Verification items for the finished model (mm, model axes). Face numbers are marked on the shaded views. A direction names the side the tool comes from. Round coordinates to 2 decimals unless told otherwise and drop trailing zeros. Order: outer loops, then holes, each group sorted by start corner. A loop starts at its lowest first (then second) coordinate and runs counter-clockwise, first axis right, second up. Notation, with made-up numbers: M -8.5,-17 L 45.5,-17 A36 cw 45.5,17 Z; hole C 10,74.25 d3. An arc over 180 degrees is marked long. Use CSV: the item, a comma, the result in double quotes. Start each with the question number.
Q1. Set-up check for the marked faces 1 and 2: record each of +Z, -Z, +X, -X, +Y, -Y from which the full face is reachable in a straight line by a thin tool's end or side.
Q2. Mould release check, pull along Y, two halves, no side actions. Record for the marked faces 3, 4, 5 and 6: +Y half, -Y half, draft (parallel to the pull), parting line (faces both ways), or undercut.
Q3. Scan lines: line 1 (Y direction, x = -143.5, z = -31.35); line 2 (Y direction, x = -143.5, z = -35.2); line 3 (X direction, y = 87, z = -26). Record each from-to range of solid material in increasing order.
Q4. Gauge pin test, flat ends, axial feed: pin 1 Ø1.5 at (y, z) = (127, -5.5) entering from +X; pin 2 Ø2 at (x, z) = (-37.5, -16.5) entering from -Y; pin 3 Ø4 at (x, y) = (-32.5, 143.5) entering from -Z. Record the tip position at first contact, or that the pin passes through.
Q5. Sectioned sample at A-A (z = -9.5). Enter the section's corners in (x, y), and give its area (3 significant figures).
Q6. Sectioned sample at B-B (y = 44). Enter the section's corners in (x, z).
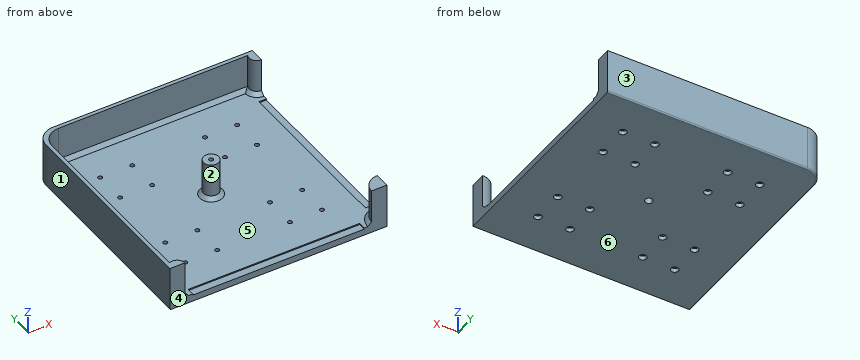
```python
from build123d import *

# Parameters (mm, degrees)
PAD005_DEPTH         = 6.25
SKETCH009_R          = 6.25
PAD006_DEPTH         = 30
SKETCH010_R          = 1.75
POCKET002_DEPTH      = 100
POCKET002_DEPTH_BACK = 100
SKETCH011_R          = 3
POCKET003_DEPTH      = 3.25
CHAMFER003_SIZE      = 3
FILLET003_R          = 1
SKETCH012_W          = 6
SKETCH012_H          = 139
SKETCH012_W_2        = 139
SKETCH012_H_2        = 6
POCKET004_DEPTH      = 1
SKETCH019_R          = 3
POCKET008_DEPTH      = 100
POCKET008_DEPTH_BACK = 24
SKETCH020_R          = 1.75
POCKET009_DEPTH      = 100
POCKET009_DEPTH_BACK = 100


with BuildPart() as part:
    # Sketch008 → Pad005 (new body)
    with BuildSketch(Plane.XY):
        with BuildLine():
            Line((88, 88), (-73.833333, 88))
            ThreePointArc((-73.833333, 88), (-83.850679, 83.850679), (-88, 73.833333))
            Line((-88, 73.833333), (-88, -88))
            Line((-88, -88), (88, -88))
            Line((88, -88), (88, 88))
        make_face()
    extrude(amount=-PAD005_DEPTH)

    # Sketch009 → Pad006 (join)
    with BuildSketch(Plane.XY):
        Circle(SKETCH009_R)
        with BuildLine():
            Line((-88, -88), (-88, 73.833333))
            ThreePointArc((-73.833333, 88), (-83.850679, 83.850679), (-88, 73.833333))
            Line((-73.833333, 88), (88, 88))
            Line((88, 88), (88, 75.889985))
            ThreePointArc((82.442769, 85), (82.664384, 78.885188), (88, 75.889985))
            Line((-70.83277, 85), (82.442769, 85))
            ThreePointArc((-70.83277, 85), (-80.85048, 80.850878), (-85, 70.833333))
            Line((-85, -82.408681), (-85, 70.833333))
            ThreePointArc((-75.957213, -88), (-78.920301, -82.684108), (-85, -82.408681))
            Line((-88, -88), (-75.957213, -88))
        make_face()
        with BuildLine():
            ThreePointArc((88, -75.5), (79.161165, -79.161165), (75.5, -88))
            Line((88, -88), (75.5, -88))
            Line((88, -88), (88, -75.5))
        make_face()
    extrude(amount=PAD006_DEPTH)

    # Sketch010 → Pocket002 (cut, two sides)
    with BuildSketch(Plane.XY) as pocket002_sk:
        with Locations((-55.5, 55.5)):
            Circle(SKETCH010_R)
        with Locations((-29.5, 55.5)):
            Circle(SKETCH010_R)
        with Locations((-29.5, 29.5)):
            Circle(SKETCH010_R)
        with Locations((-55.5, 29.5)):
            Circle(SKETCH010_R)
        with Locations((29.5, 55.5)):
            Circle(SKETCH010_R)
        with Locations((55.5, 55.5)):
            Circle(SKETCH010_R)
        with Locations((55.5, 29.5)):
            Circle(SKETCH010_R)
        with Locations((29.5, 29.5)):
            Circle(SKETCH010_R)
        with Locations((29.5, -29.5)):
            Circle(SKETCH010_R)
        with Locations((55.5, -29.5)):
            Circle(SKETCH010_R)
        with Locations((55.5, -55.5)):
            Circle(SKETCH010_R)
        with Locations((29.5, -55.5)):
            Circle(SKETCH010_R)
        with Locations((-55.5, -29.5)):
            Circle(SKETCH010_R)
        with Locations((-29.5, -29.5)):
            Circle(SKETCH010_R)
        with Locations((-29.5, -55.5)):
            Circle(SKETCH010_R)
        with Locations((-55.5, -55.5)):
            Circle(SKETCH010_R)
    extrude(amount=-POCKET002_DEPTH, mode=Mode.SUBTRACT)
    extrude(pocket002_sk.sketch, amount=POCKET002_DEPTH_BACK, mode=Mode.SUBTRACT)

    # Sketch011 → Pocket003 (cut)
    with BuildSketch(Plane.XY.offset(-6.25)):
        with Locations((-55.5, 55.5)):
            Circle(SKETCH011_R)
        with Locations((-29.5, 55.5)):
            Circle(SKETCH011_R)
        with Locations((-29.5, 29.5)):
            Circle(SKETCH011_R)
        with Locations((-55.5, 29.5)):
            Circle(SKETCH011_R)
        with Locations((29.5, 55.5)):
            Circle(SKETCH011_R)
        with Locations((55.5, 55.5)):
            Circle(SKETCH011_R)
        with Locations((55.5, 29.5)):
            Circle(SKETCH011_R)
        with Locations((29.5, 29.5)):
            Circle(SKETCH011_R)
        with Locations((29.5, -29.5)):
            Circle(SKETCH011_R)
        with Locations((55.5, -29.5)):
            Circle(SKETCH011_R)
        with Locations((55.5, -55.5)):
            Circle(SKETCH011_R)
        with Locations((29.5, -55.5)):
            Circle(SKETCH011_R)
        with Locations((-55.5, -29.5)):
            Circle(SKETCH011_R)
        with Locations((-29.5, -29.5)):
            Circle(SKETCH011_R)
        with Locations((-29.5, -55.5)):
            Circle(SKETCH011_R)
        with Locations((-55.5, -55.5)):
            Circle(SKETCH011_R)
    extrude(amount=POCKET003_DEPTH, mode=Mode.SUBTRACT)

    # Chamfer003
    chamfer003_edges = [part.edges().sort_by_distance(p)[0] for p in [
        (-6.25, 0, 0),
        (79.161165, -79.161165, 0),
        (82.664384, 78.885188, 0),
        (-78.920301, -82.684108, 0),
        (5.804999, 85, 0),
    ]]
    chamfer(chamfer003_edges, length=CHAMFER003_SIZE)

    # Fillet003
    fillet003_edges = [part.edges().sort_by_distance(p)[0] for p in [
        (-88, -7.083333, -6.25),
    ]]
    fillet(fillet003_edges, radius=FILLET003_R)

    # Sketch012 → Pocket004 (cut)
    with BuildSketch(Plane.XY):
        with Locations((85, 0)):
            Rectangle(SKETCH012_W, SKETCH012_H)
        with Locations((0, -85)):
            Rectangle(SKETCH012_W_2, SKETCH012_H_2)
    extrude(amount=-POCKET004_DEPTH, mode=Mode.SUBTRACT)

    # Sketch019 → Pocket008 (cut, two sides)
    with BuildSketch(Plane.XY) as pocket008_sk:
        Circle(SKETCH019_R)
    extrude(amount=-POCKET008_DEPTH, mode=Mode.SUBTRACT)
    extrude(pocket008_sk.sketch, amount=POCKET008_DEPTH_BACK, mode=Mode.SUBTRACT)

    # Sketch020 → Pocket009 (cut, two sides)
    with BuildSketch(Plane.XY) as pocket009_sk:
        Circle(SKETCH020_R)
    extrude(amount=-POCKET009_DEPTH, mode=Mode.SUBTRACT)
    extrude(pocket009_sk.sketch, amount=POCKET009_DEPTH_BACK, mode=Mode.SUBTRACT)


with BuildPart() as part_1:
    # Body002 placement: moved
    add(part.part.moved(Location((-88, 88, -30))))


solid = part_1.part
```
Verdict:
1,face 1,"+Z, -Z, -X, +Y, -Y"
1,face 2,"+Z"
2,face 3,"+Y half"
2,face 4,"-Y half"
2,face 5,"undercut"
2,face 6,"draft"
3,line 1,"y = 0 to 30.75, 34.25 to 56.75, 60.25 to 115.75, 119.25 to 141.75, 145.25 to 176"
3,line 2,"y = 0 to 29.5, 35.5 to 55.5, 61.5 to 114.5, 120.5 to 140.5, 146.5 to 176"
3,line 3,"x = -176 to -173, -94.17 to -90.83, -85.17 to -81.83"
4,pin 1,"stops at x = -173"
4,pin 2,"stops at y = 173"
4,pin 3,"stops at z = -33"
5,outline,"M -176,0 L -163.96,0 A6.25 ccw -173,5.59 L -173,158.83 A14.17 cw -158.83,173 L -5.56,173 A6.25 ccw 0,163.89 L 0,176 L -161.83,176 A14.17 ccw -176,161.83 Z; C -88,88 d12.5; M -12.5,0 L 0,0 L 0,12.5 A12.5 ccw Z; hole C -88,88 d6"
5,area,"1,360 mm²"
6,outline,"M -176,-35.25 A1 ccw -175,-36.25 L 0,-36.25 L 0,-31 L -6,-31 L -6,-30 L -170,-30 L -173,-27 L -173,0 L -176,0 Z"
